```python
from build123d import *

# Parameters (mm, degrees)
SKETCH1_R               = 88.9
BOSS_EXTRUDE1_DEPTH     = 9.525
SKETCH2_R               = 45.72
CUT_EXTRUDE1_DEPTH      = 12.7
SKETCH3_R               = 1.143
CUT_EXTRUDE2_DEPTH      = 12.7
CUT_EXTRUDE3_DEPTH      = 127.083883288
CUT_EXTRUDE3_DEPTH_BACK = 127.083883288
CIRPATTERN1_COUNT       = 12
SKETCH6_R               = 1.143
CUT_EXTRUDE4_DEPTH      = 25.4
SKETCH7_R               = 0.6985
CUT_EXTRUDE5_DEPTH      = 3.175
CIRPATTERN2_COUNT       = 4


with BuildPart() as part:
    # Sketch1 → Boss-Extrude1 (new body)
    with BuildSketch(Plane(origin=(0, 0, 0), x_dir=(1, 0, 0), z_dir=(0, 1, 0))):
        with Locations(Location((0, 0, 0), (0, 0, 90))):
            Circle(SKETCH1_R)
    extrude(amount=BOSS_EXTRUDE1_DEPTH)

    # Sketch2 → Cut-Extrude1 (cut)
    with BuildSketch(Plane(origin=(0, 9.525, 0), x_dir=(1, 0, 0), z_dir=(0, 1, 0))):
        with Locations(Location((0, 0, 0), (0, 0, 270))):
            Circle(SKETCH2_R)
    extrude(amount=-CUT_EXTRUDE1_DEPTH, mode=Mode.SUBTRACT)

    # Sketch3 → Cut-Extrude2 (cut)
    with BuildSketch(Plane(origin=(0, 9.525, 0), x_dir=(1, 0, 0), z_dir=(0, 1, 0))):
        with Locations(Location((13.364949615, 49.878671003, 0), (0, 0, 270))):
            Circle(SKETCH3_R)
    cut_extrude2 = extrude(amount=-CUT_EXTRUDE2_DEPTH, mode=Mode.SUBTRACT)

    # Sketch5 → Cut-Extrude3 (cut, two sides)
    with BuildSketch(Plane(origin=(0, 9.525, 0), x_dir=(1, 0, 0), z_dir=(0, 1, 0))) as cut_extrude3_sk:
        Polygon((0, 139.125590331), (0, -130.538836117), (-200.055019192, 4.293377107), align=None)
    extrude(amount=CUT_EXTRUDE3_DEPTH, mode=Mode.SUBTRACT)
    extrude(cut_extrude3_sk.sketch, amount=-CUT_EXTRUDE3_DEPTH_BACK, mode=Mode.SUBTRACT)

    # CirPattern1: Cut-Extrude2 ×12 about axis
    cirpattern1_axis = Axis((0, 9.525, 0), (0, 1, 0))
    for i in range(1, CIRPATTERN1_COUNT):
        add(cut_extrude2.rotate(cirpattern1_axis, i * 360 / CIRPATTERN1_COUNT), mode=Mode.SUBTRACT)

    # Sketch6 → Cut-Extrude4 (cut)
    with BuildSketch(Plane(origin=(88.9, 0, 0), x_dir=(0, 0, -1), z_dir=(1, 0, 0))):
        with Locations((0, 4.826)):
            Circle(SKETCH6_R)
    extrude(amount=-CUT_EXTRUDE4_DEPTH, mode=Mode.SUBTRACT)

    # Sketch7 → Cut-Extrude5 (cut)
    with BuildSketch(Plane(origin=(62.861792847, 0, 62.861792847), x_dir=(0, -1, 0), z_dir=(0.7071067811865464, 0, 0.7071067811865488))):
        with Locations(Location((-4.826, 0, 0), (0, 0, 90))):
            Circle(SKETCH7_R)
    cut_extrude5 = extrude(amount=-CUT_EXTRUDE5_DEPTH, mode=Mode.SUBTRACT)

    # CirPattern2: Cut-Extrude5 ×4 about axis
    cirpattern2_axis = Axis((0, 9.525, 0), (0, 1, 0))
    for i in range(1, CIRPATTERN2_COUNT):
        add(cut_extrude5.rotate(cirpattern2_axis, i * 360 / CIRPATTERN2_COUNT), mode=Mode.SUBTRACT)


solid = part.part
```
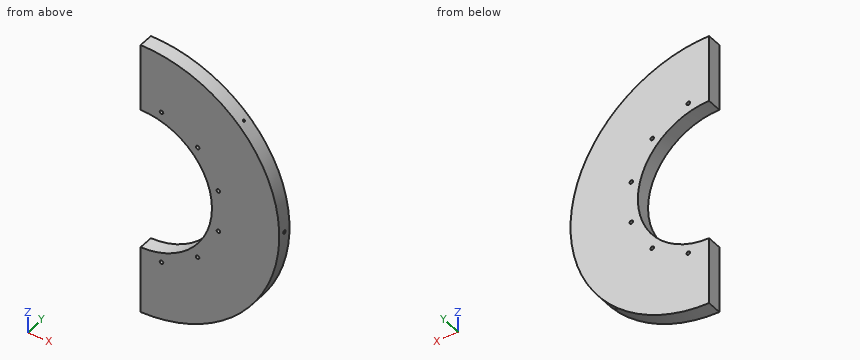
Input: part model. Units: mm. Frame: model coordinates. Coordinates: 2 decimals unless noted, no trailing zeros. Write each loop counter-clockwise with the first axis right and the second up, starting at its lowest first coordinate (ties: lowest second). Pieces come first, ordered by that corner, then holes. Notation, with made-up numbers: (-21.75, 28.5) -> (21.25, 28.5) arc R16 cw to (21.25, 37.5) -> close; hole circle Ø2 at (74, 54). An arc over 180 degrees is marked (long way). Answer as a JSON object with one key per item and string values.
1. Section B-B on y = 1.5. Return the cut outline in (x, z), then the cut area to 3 significant figures.
Result set:
{"outline": "(0, -88.9) arc R88.9 ccw to (0, 88.9) -> (0, 45.72) arc R45.72 cw to (0, -45.72) -> close; hole circle Ø2.29 at (13.36, -49.88); hole circle Ø2.29 at (13.36, 49.88); hole circle Ø2.29 at (36.51, -36.51); hole circle Ø2.29 at (36.51, 36.51); hole circle Ø2.29 at (49.88, -13.36); hole circle Ø2.29 at (49.88, 13.36)", "area": "9,110 mm2"}
2. Material intervals for line 1 (Z direction, x = 49, y = 5.5); line 2 (Z direction, x = 14, y = 4.5); line 3 (Z direction, x = 25, y = 0.5), sorted ascending. Write a range as from..to.
Result set:
{"line 1": "z = -74.18..-14.1, -12.63..12.63, 14.1..74.18", "line 2": "z = -87.79..-50.83, -48.93..-43.52, 43.52..48.93, 50.83..87.79", "line 3": "z = -85.31..-38.28, 38.28..85.31"}
3. First-contact query: P1, Ø1, axis at y = 4.5, z = 19.5, coming from the -X side; P2, Ø2, axis at y = 4.826, z = 0, coming from the +X side; P3, Ø1, axis at x = 70, y = 6.5, coming from the +Z side. Flat tips, straight axial feed; report the tip coordinate or a pass-through.
Result set:
{"P1": "stops at x = 41.11", "P2": "stops at x = 63.5", "P3": "stops at z = 55.43"}
4. Section A-A on x = 83. Return the cut outline in (y, z) (3 decimals), then the cut area to 3 significant figures.
Result set:
{"outline": "(0, -31.847) -> (9.525, -31.847) -> (9.525, 31.847) -> (0, 31.847) -> close; hole circle Ø2.286 at (4.826, 0)", "area": "603 mm2"}
5. Section C-C on z = -7.5. Return the cut outline in (x, y) (3 decimals).
Result set:
{"outline": "(45.101, 0) -> (88.583, 0) -> (88.583, 9.525) -> (45.101, 9.525) -> close"}
6. Section D-D on x = 72. Return the cut outline in (y, z) (3 decimals), then the cut area to 3 significant figures.
Result set:
{"outline": "(0, -52.146) -> (9.525, -52.146) -> (9.525, 52.146) -> (0, 52.146) -> close; hole circle Ø2.286 at (4.826, 0)", "area": "989 mm2"}
